Read the model definition and answer for the solid it produces. Units are mm, in the model's axes. Give positions to 0.01 mm unless a question says otherwise; leave off trailing zeros. Order: outer loops, then holes, each group sorted by start corner. A loop starts at its lowest first (then second) coordinate and runs counter-clockwise, first axis right, second up. Notation, with made-up numbers: (89.5, -39.5) -> (93.5, -39.5) arc R11 cw to (93.5, -22.5) -> close; hole circle Ø10 at (40, -0.75). An arc over 180 degrees is marked (long way). Use one line per item in the form item = value.
Autodesk Inventor part; units mm, degrees
ref_plane "YZ Plane" through (0, 0, 0) normal (1, 0, 0) x (0, 1, 0)
ref_plane "XZ Plane" through (0, 0, 0) normal (0, 1, 0) x (-1, 0, 0)
ref_plane "XY Plane" through (0, 0, 0) normal (0, 0, 1) x (1, 0, 0)
sketch "Sketch1" plane through (0, 0, 0) normal (0, 1, 0) x (-1, 0, 0)
  line L0 (0, 0) -> (138.2, 0)
  line L1 (138.2, 0) -> (138.2, -72.8)
  line L2 (138.2, -72.8) -> (0, -72.8)
  line L3 (0, -72.8) -> (0, 0)
  dimension "d0" = 138.2
  dimension "d1" = 72.8
extrude "Extrusion1" add sketch "Sketch1" along normal blind 1.3
sketch "Sketch2" plane through (0, 1.3, 0) normal (0, 1, 0) x (1, 0, 0)
  line L0 (0, 72.8) -> (-138.2, 72.8)
  line L1 (0, 72.8) -> (-100, 72.8)
  line L2 (-100, 72.8) -> (-100, 46.3)
  circle A0 centre (-100, 46.3) radius 1.65
  point P0 (0, 0)
  dimension "d4" = 100
  dimension "d5" = 26.5
  dimension "d6" = 3.3
extrude "Extrusion2" cut sketch "Sketch2" against normal through all
sketch "Sketch3" plane through (0, 1.3, 0) normal (0, 1, 0) x (1, 0, 0)
  line L0 (-138.2, 0) -> (0, 0)
  line L1 (0, 0) -> (0, 10)
  line L2 (0, 0) -> (0, 72.8)
  line L3 (0, 10) -> (-10, 10)
  line L4 (0, 72.8) -> (0, 62.8)
  line L5 (0, 62.8) -> (-10, 62.8)
  line L6 (-10, 10) -> (-13, 10)
  line L7 (-13, 10) -> (-13, 62.8)
  line L8 (-13, 62.8) -> (-10, 62.8)
  line L9 (-10, 62.8) -> (-10, 10)
  dimension "d9" = 10
  dimension "d10" = 10
  dimension "d11" = 10
  dimension "d12" = 10
  dimension "d13" = 3
extrude "Extrusion3" add sketch "Sketch3" along normal blind 1.6 contours L6 L7 L8 L9
properties part number "Lid_3DPrint"
Item 1: Given pin 1 Ø1.3 at (y, z) = (2.5, -33) entering from -X; pin 2 Ø1.3 at (x, y) = (-12, 2) entering from -Z; pin 3 Ø1.5 at (x, z) = (-90, -12.5) entering from +Y, each flat-ended and moving along its own axis, determine where each tip first touches the part or whether it passes through.
Checks:
pin_1 = -13
pin_2 = -62.8
pin_3 = 1.3
Item 2: The part is cut by section D-D on x = -56. Give the vertices of the cut face in (y, z), and give its area (3 significant figures).
Checks:
outline = (0, -72.8) -> (1.3, -72.8) -> (1.3, 0) -> (0, 0) -> close
area = 94.6 mm²
Item 3: The part is cut by section B-B on z = -46.3. Give the vertices of the cut face in (x, y).
Checks:
outline = (-138.2, 0) -> (-101.65, 0) -> (-101.65, 1.3) -> (-138.2, 1.3) -> close; (-98.35, 0) -> (0, 0) -> (0, 1.3) -> (-10, 1.3) -> (-10, 2.9) -> (-13, 2.9) -> (-13, 1.3) -> (-98.35, 1.3) -> close
Item 4: The part is cut by section C-C on z = -15.5. Give the vertices of the cut face in (x, y).
Checks:
outline = (-138.2, 0) -> (0, 0) -> (0, 1.3) -> (-10, 1.3) -> (-10, 2.9) -> (-13, 2.9) -> (-13, 1.3) -> (-138.2, 1.3) -> close
Item 5: The part is cut by section A-A on x = -100. Give the vertices of the cut face in (y, z), and give its area (4 significant figures).
Checks:
outline = (0, -72.8) -> (1.3, -72.8) -> (1.3, -47.95) -> (0, -47.95) -> close; (0, -44.65) -> (1.3, -44.65) -> (1.3, 0) -> (0, 0) -> close
area = 90.35 mm²
Item 6: Determine the mould class of faces 1 (the flat face through (-12, 2.9, -37)), 2 (the cylindrical face through (-101.65, 0.66, -46.37)) for opening direction X: +X half, -X half, draft (parallel to the pull), parting line (faces both ways), or undercut.
Checks:
face_1 = draft
face_2 = undercut
Item 7: Straight lines are drawn through the part: L1, parallel to X at y = 0.4, z = -46.3; L2, parallel to Z at x = -100, y = 0.75; L3, parallel to Y at x = -121, z = -6. For each, find the intervals that lie inside material, in ascending order. Write a range as from..to.
Checks:
L1 = -138.2..-101.65, -98.35..0
L2 = -72.8..-47.95, -44.65..0
L3 = 0..1.3
